```python
from build123d import *

# Parameters (mm, degrees)
SKETCH1_R           = 2.2
BOSS_EXTRUDE1_DEPTH = 3.9
BOSS_EXTRUDE2_START = -2
SKETCH1_4_R         = 2.2
BOSS_EXTRUDE2_DEPTH = 2


with BuildPart() as part:
    # Sketch1 → Boss-Extrude1 (new body)
    with BuildSketch(Plane.XY):
        with BuildLine():
            Line((1, 0), (22, 0))
            ThreePointArc((22, 0), (22.707106781, 0.292893219), (23, 1))
            Line((23, 1), (23, 8))
            Line((23, 8), (0, 8))
            Line((0, 8), (0, 1))
            ThreePointArc((0, 1), (0.292893219, 0.292893219), (1, 0))
        make_face()
        with Locations((19, 3)):
            Circle(SKETCH1_R, mode=Mode.SUBTRACT)
        with Locations((4, 3)):
            Circle(SKETCH1_R, mode=Mode.SUBTRACT)
    extrude(amount=BOSS_EXTRUDE1_DEPTH)

    # Sketch1<4> → Boss-Extrude2 (add)
    with BuildSketch(Plane.XY.offset(BOSS_EXTRUDE2_START)):
        with BuildLine():
            Line((-0.8, 8.8), (-0.8, 1))
            ThreePointArc((-0.8, 1), (-0.272792206, -0.272792206), (1, -0.8))
            Line((1, -0.8), (22, -0.8))
            ThreePointArc((22, -0.8), (23.272792206, -0.272792206), (23.8, 1))
            Line((23.8, 1), (23.8, 8.8))
            Line((23.8, 8.8), (-0.8, 8.8))
        make_face()
        with Locations((4, 3)):
            Circle(SKETCH1_4_R, mode=Mode.SUBTRACT)
        with Locations((19, 3)):
            Circle(SKETCH1_4_R, mode=Mode.SUBTRACT)
    extrude(amount=BOSS_EXTRUDE2_DEPTH)


solid = part.part
```
Geometry: final body of the model. Coordinates: model frame, mm. A direction names the side the tool comes from. Give positions to 0.01 mm unless a question says otherwise; leave off trailing zeros. Loops run counter-clockwise (first coordinate to the right, second up) from the corner with the lowest first, then second, coordinate; pieces in that order, holes last. Notation, with made-up numbers: (70, -6.5) - (101, -6.5) arc R15 cw to (101, 18.5) - close; hole circle Ø7 at (-28.75, 55). An arc over 180 degrees is marked (long way). Answer as CSV lines item,"result". Start each with the question number.
(1) Pin query (flat end, axial travel): P1, Ø1.2, axis at x = 13.5, z = 2.5, coming from the +Y side; P2, Ø3, axis at y = 6, z = 2.5, coming from the +X side. Return the tip coordinate at first contact, or that it passes through.
(2) Ray query, line 1 along X through (y, z) = (1, -0.1); line 2 along Y through (x, z) = (4, 0.45); line 3 along X through (y, z) = (3.75, 0.5). Return the intervals inside material, ascending. Write a range as [from, to].
(3) Section query A-A (y = 3). Output: boundary loops of the cut face in (x, z).
(4) Reachability of faces 1 (the face through (12, 8, 2)), 2 (the face through (0.285, 0.301, 1.923)), 3 (the face through (11, 0, 2)), 4 (the face through (22.699, 0.285, 1.923)) from +Z, -Z, +X, -X, +Y, -Y: full face, straight path, thin tool, end or side. Return the list, or none.
(5) Section query C-C (z = 1.75). Output: boundary loops of the cut face in (x, y).
(6) Mould query, pull axis X, two halves, no side actions, for faces 5 (the face through (5.183, 4.855, 0.909)), 6 (the face through (23, 4, 2)), 7 (the face through (0, 5, 2)), 8 (the face through (12, 8.8, -1)). Classes: +X half, -X half, draft (parallel to the pull), parting line (faces both ways), or undercut.
(7) Section query D-D (x = 11.5). Output: boundary loops of the cut face in (y, z).
(8) Section query B-B (x = 19). Output: boundary loops of the cut face in (y, z), and give its area (3 significant figures).
Worked answers:
1,P1,"stops at y = 8"
1,P2,"stops at x = 23"
2,line 1,"x = [-0.8, 3.08], [4.92, 18.08], [19.92, 23.8]"
2,line 2,"y = [0, 0.8], [5.2, 8]"
2,line 3,"x = [0, 1.93], [6.07, 16.93], [21.07, 23]"
3,outline,"(-0.8, -2) - (1.8, -2) - (1.8, 3.9) - (0, 3.9) - (0, 0) - (-0.8, 0) - close; (6.2, -2) - (16.8, -2) - (16.8, 3.9) - (6.2, 3.9) - close; (21.2, -2) - (23.8, -2) - (23.8, 0) - (23, 0) - (23, 3.9) - (21.2, 3.9) - close"
4,face 1,"+Z, +X, -X, +Y"
4,face 2,"+Z, -X, -Y"
4,face 3,"+Z, +X, -X, -Y"
4,face 4,"+Z, +X, -Y"
5,outline,"(0, 1) arc R1 ccw to (1, 0) - (22, 0) arc R1 ccw to (23, 1) - (23, 8) - (0, 8) - close; hole circle Ø4.4 at (4, 3); hole circle Ø4.4 at (19, 3)"
6,face 5,"undercut"
6,face 6,"+X half"
6,face 7,"-X half"
6,face 8,"draft"
7,outline,"(-0.8, -2) - (8.8, -2) - (8.8, 0) - (8, 0) - (8, 3.9) - (0, 3.9) - (0, 0) - (-0.8, 0) - close"
8,outline,"(-0.8, -2) - (0.8, -2) - (0.8, 3.9) - (0, 3.9) - (0, 0) - (-0.8, 0) - close; (5.2, -2) - (8.8, -2) - (8.8, 0) - (8, 0) - (8, 3.9) - (5.2, 3.9) - close"
8,area,"24.4 mm^2"
